The listing builds one solid part. Answer for the finished solid, in the listing's coordinates (mm). A direction names the side the tool comes from. Give positions to 0.01 mm unless a question says otherwise; leave off trailing zeros. Loops run counter-clockwise (first coordinate to the right, second up) from the corner with the lowest first, then second, coordinate; pieces in that order, holes last. Notation, with made-up numbers: (78.5, -1) - (93.5, -1) arc R28 cw to (93.5, 32) - close; hole circle Ø10 at (4, -24.5). An arc over 180 degrees is marked (long way). Write item = value, one per line. Start each with the question number.
1) Which of the six approach directions +Z, -Z, +X, -X, +Y, -Y give full straight-line access (tool end or side, diameter ignored) to faces 1 (the cylindrical face through (-206.35, -6.26, 102.01)), 2 (the flat face through (-127, -3.175, 28))?
2) The part is cut by section A-A on x = -50.8. Write down the section's boundary in (y, z) (3 decimals), plus the area to 3 significant figures.
3) Flat-ended cylindrical pins translate along their axes: P1, Ø4, axis at x = -50.8, z = 101.6, coming from the -Y side; P2, Ø10, axis at x = -127.5, z = 61, coming from the +Y side; P3, Ø17, axis at x = -137, z = 39.5, coming from the +Y side (3 decimals). Find the tip coordinate at first contact, or state that the pin passes through.
4) The mould has two halves that part along X. Classify faces 3 (the flat face through (-125, -6, 0)), 4 (the cylindrical face through (-53.95, -6.26, 102.01)), 5 (the flat face through (-254, -6, 75)): +X half, -X half, draft (parallel to the pull), parting line (faces both ways), or undercut.
5) The part is cut by section B-B on x = -127. Write down the section's boundary in (y, z) (3 decimals), plus the area to 3 significant figures.
6) Consider probe 1 along Z at (x, y) = (-127, -8.75) (3 decimals); probe 2 along Z at (x, y) = (-127, -3.7) (3 decimals); probe 3 along Z at (x, y) = (-106, -3). Determine where each line is inside the solid, lowest interval first.
Autodesk Inventor part; units mm, degrees
ref_plane "YZ Plane" through (0, 0, 0) normal (1, 0, 0) x (0, 1, 0)
ref_plane "XZ Plane" through (0, 0, 0) normal (0, 1, 0) x (-1, 0, 0)
ref_plane "XY Plane" through (0, 0, 0) normal (0, 0, 1) x (1, 0, 0)
sketch "Sketch1" plane through (0, 0, 0) normal (0, 1, 0) x (-1, 0, 0)
  line L0 (0, 0) -> (254, 0)
  line L1 (254, 0) -> (254, 152.4)
  line L2 (254, 152.4) -> (0, 152.4)
  line L3 (0, 152.4) -> (0, 0)
  dimension "d0" = 254
  dimension "d1" = 152.4
extrude "Extrusion1" add sketch "Sketch1" against normal blind 12.7
sketch "Sketch2" plane through (0, 0, 0) normal (0, 1, 0) x (1, 0, 0)
  line L0 (0, 0) -> (-254, 0)
  line L1 (-254, 0) -> (-254, -152.4)
  line L2 (0, -152.4) -> (0, 0)
  line L3 (-155.575, -19.05) -> (-98.425, -19.05)
  line L4 (-98.425, -19.05) -> (-98.425, -76.2)
  line L5 (-98.425, -76.2) -> (-155.575, -76.2)
  line L6 (-155.575, -76.2) -> (-155.575, -19.05)
  dimension "d4" = 57.15
  dimension "d6" = 57.15
  dimension "d7" = 98.425
  dimension "d8" = 98.425
  dimension "d9" = 19.05
extrude "Extrusion2" cut sketch "Sketch2" against normal blind 3.175
sketch "Sketch3" plane through (0, -3.175, 0) normal (0, 1, 0) x (1, 0, 0)
  line L0 (-98.425, -76.2) -> (-155.575, -76.2)
  line L1 (-98.425, -19.05) -> (-98.425, -76.2)
  circle A0 centre (-127, -47.625) radius 19.05
  point P0 (0, 0)
  dimension "d12" = 38.1
  dimension "d13" = 28.575
  dimension "d14" = 28.575
extrude "Extrusion3" cut sketch "Sketch3" against normal blind 1.524
sketch "Sketch4" plane through (-127, -4.699, 47.625) normal (0, 1, 0) x (1, 0, 0)
  circle A0 centre (0, 0) radius 19.05
  circle A1 centre (0, 0) radius 3.81
  point P0 (127, 47.625)
  dimension "d17" = 7.62
extrude "Extrusion4" cut sketch "Sketch4" against normal through all contours A1
sketch "Sketch5" plane through (0, -12.7, 0) normal (0, -1, 0) x (1, 0, 0)
  line L0 (0, 0) -> (0, 152.4)
  line L1 (0, 152.4) -> (-254, 152.4)
  line L2 (-254, 152.4) -> (-254, 0)
  circle A0 centre (-127, 47.625) radius 3.81
  point P0 (-50.8, 101.6)
  point P1 (-203.2, 101.6)
  point P2 (-127, 106.68)
  dimension "d20" = 50.8
  dimension "d21" = 50.8
  dimension "d22" = 50.8
  dimension "d30" = 5.08
hole "Hole1" at (-50.8, -12.7, 101.6) at (-203.2, -12.7, 101.6) at (-127, -12.7, 106.68) direction (0, 1, 0) diameter 6.35 end through all
equation "\"d7\" = d8"
properties part number "tractor"
Answer below:
q1.face_1 = +Y, -Y
q1.face_2 = +Y
q2.outline = (-12.7, 0) - (0, 0) - (0, 98.425) - (-12.7, 98.425) - close; (-12.7, 104.775) - (0, 104.775) - (0, 152.4) - (-12.7, 152.4) - close
q2.area = 1,850 mm2
q3.P1 = through
q3.P2 = -4.7
q3.P3 = -3.175
q4.face_3 = draft
q4.face_4 = undercut
q4.face_5 = -X half
q5.outline = (-12.7, 0) - (0, 0) - (0, 19.05) - (-3.175, 19.05) - (-3.175, 28.575) - (-4.699, 28.575) - (-4.699, 43.815) - (-12.7, 43.815) - close; (-12.7, 51.435) - (-4.699, 51.435) - (-4.699, 66.675) - (-3.175, 66.675) - (-3.175, 76.2) - (0, 76.2) - (0, 103.505) - (-12.7, 103.505) - close; (-12.7, 109.855) - (0, 109.855) - (0, 152.4) - (-12.7, 152.4) - close
q5.area = 1,550 mm2
q6.probe_1 = 0 to 43.815, 51.435 to 103.505, 109.855 to 152.4
q6.probe_2 = 0 to 28.575, 66.675 to 103.505, 109.855 to 152.4
q6.probe_3 = 0 to 19.05, 76.2 to 152.4
